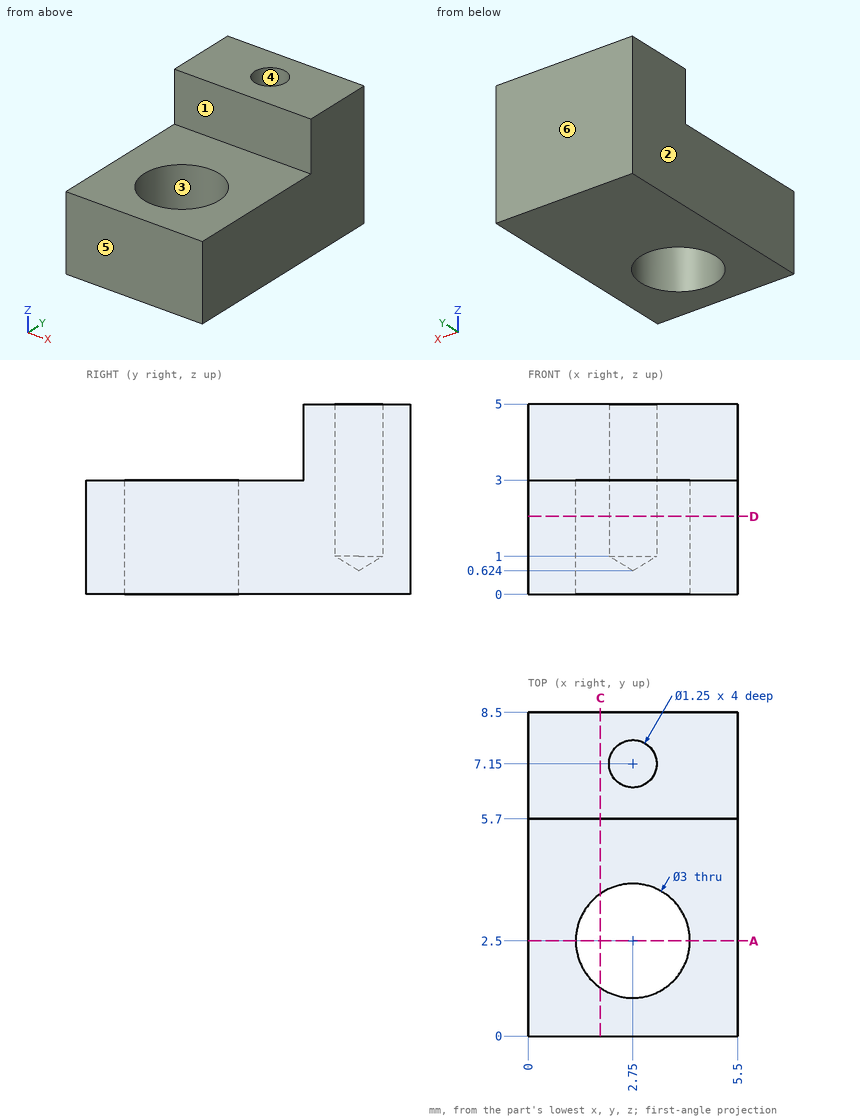
Verification items for this drawing (mm, ordinates from the low corner). A direction names the side the tool comes from. Give positions to 0.01 mm unless a question says otherwise; leave off trailing zeros. Write each loop counter-clockwise with the first axis right and the second up, starting at its lowest first coordinate (ties: lowest second). Pieces come first, ordered by that corner, then holes. Notation, with made-up numbers: (45.25, -17) -> (67.25, -17) arc R8 ccw to (67.25, -6) -> close; hole circle Ø1 at (84.25, 28.25). An arc over 180 degrees is marked (long way). Use one line per item in the form item = value.
Item 1: Sectioned sample at A-A on y = 2.5. Enter the section's corners in (x, z).
Results list:
outline = (0, 0) -> (1.25, 0) -> (1.25, 3) -> (0, 3) -> close; (4.25, 0) -> (5.5, 0) -> (5.5, 3) -> (4.25, 3) -> close
Item 2: Sectioned sample at C-C on x = 1.9. Enter the section's corners in (y, z) (1 decimal).
Results list:
outline = (0, 0) -> (1.3, 0) -> (1.3, 3) -> (0, 3) -> close; (3.7, 0) -> (8.5, 0) -> (8.5, 5) -> (5.7, 5) -> (5.7, 3) -> (3.7, 3) -> close
Item 3: Depth check by flat-ended pin: pin 1 Ø1 at (x, z) = (1.5, 2) entering from -Y; pin 2 Ø3 at (x, y) = (2.5, 1.5) entering from +Z; pin 3 Ø2 at (x, z) = (3, 4.5) entering from -Y. Enter the tip coordinate at first touch or a pass-through.
Results list:
pin_1 = 0
pin_2 = 3
pin_3 = 5.7
Item 4: Scan lines: line 1 (Y direction, x = 2.75, z = 2.75) (1 decimal); line 2 (Y direction, x = 2.75, z = 3.65) (1 decimal); line 3 (X direction, y = 7.15, z = 2.4) (1 decimal). Record each from-to range of solid material in increasing order.
Results list:
line_1 = 0 to 1, 4 to 6.5, 7.8 to 8.5
line_2 = 5.7 to 6.5, 7.8 to 8.5
line_3 = 0 to 2.1, 3.4 to 5.5
Item 5: Sectioned sample at D-D on z = 2.05. Count the separate pieces of the cut face and the enclosed holes in it.
Results list:
separate_pieces = 1
enclosed_holes = 2
Item 6: Access from +Z, -Z, +X, -X, +Y, -Y to the whole of each face (thin tool, end or side, straight path). Record for the marked faces 1 and 2.
Results list:
face_1 = +Z, +X, -X, -Y
face_2 = +Z, -Z, -X, +Y, -Y
Item 7: Mould release check, pull along Y, two halves, no side actions. Record for the marked faces 3, 4, 5 and 6: released by +Y, released by -Y, zero draft, split by the parting line, or undercut.
Results list:
face_3 = undercut
face_4 = undercut
face_5 = released by -Y
face_6 = released by +Y
